```python
from build123d import *

# Parameters (mm, degrees)
F0_W      = 60
F0_H      = 60
F0_R      = 1.665
F1_DEPTH  = 5
F2_W      = 60
F2_H      = 20
F3_DEPTH  = 5
F5_DEPTH  = 5
F7_R      = 1.945
F8_DEPTH  = 5
F9_R      = 12.55
F10_DEPTH = 2


with BuildPart() as f1:
    # F0 (on Top) → F1 (new body)
    with BuildSketch(Plane.XY):
        Rectangle(F0_W, F0_H)
        with Locations((-15, -15)):
            Circle(F0_R, mode=Mode.SUBTRACT)
        with Locations((15, -15)):
            Circle(F0_R, mode=Mode.SUBTRACT)
        with Locations((-15, 15)):
            Circle(F0_R, mode=Mode.SUBTRACT)
        with Locations((15, 15)):
            Circle(F0_R, mode=Mode.SUBTRACT)
    extrude(amount=F1_DEPTH)

    # F2 (on face) → F3 (join)
    with BuildSketch(Plane.XZ.offset(30)):
        with Locations((0, -5)):
            Rectangle(F2_W, F2_H)
    extrude(amount=F3_DEPTH)

    # F4 (on face) → F5 (join)
    with BuildSketch(Plane.YZ.offset(30)):
        Polygon((-30, -15), (30, 0), (30, 5), (-35, 5), (-35, -15), align=None)
    extrude(amount=F5_DEPTH)

    # F6: F1 across plane


with BuildPart() as f1_1:
    add(f1.part)
    add(f1.part.mirror(Plane.YZ))

    # F7 (on face) → F8 (cut, through all)
    with BuildSketch(Plane.XZ.offset(35)):
        with Locations((-25, -5)):
            Circle(F7_R)
        with Locations((25, -5)):
            Circle(F7_R)
    extrude(amount=-F8_DEPTH, mode=Mode.SUBTRACT)

    # F9 (on face) → F10 (cut)
    with BuildSketch(Plane.XY.offset(5)):
        with Locations((0, 3.7)):
            Circle(F9_R)
    extrude(amount=-F10_DEPTH, mode=Mode.SUBTRACT)


solid = f1_1.part
```
Input: part model. Units: mm. Frame: model coordinates. A direction names the side the tool comes from. Round coordinates to 2 decimals unless told otherwise and drop trailing zeros. Write each loop counter-clockwise with the first axis right and the second up, starting at its lowest first coordinate (ties: lowest second). Pieces come first, ordered by that corner, then holes. Notation, with made-up numbers: (45, 18) - (89, 18) arc R18 cw to (89, 50) - close; hole circle Ø9 at (37, 27.5). An arc over 180 degrees is marked (long way). Write item = value, one per line.
(1) Section query C-C on z = -9.25. Output: boundary loops of the cut face in (x, y).
Geometry check:
outline = (-35, -35) - (35, -35) - (35, -7) - (30, -7) - (30, -30) - (-30, -30) - (-30, -7) - (-35, -7) - close
(2) Section query A-A on x = -25. Output: boundary loops of the cut face in (y, z) (3 decimals), then the cut area to 3 significant figures.
Geometry check:
outline = (-35, -15) - (-30, -15) - (-30, -6.945) - (-35, -6.945) - close; (-35, -3.055) - (-30, -3.055) - (-30, 0) - (30, 0) - (30, 5) - (-35, 5) - close
area = 381 mm^2
(3) Contact query for flat-ended pins moving along their axis: pin 1 Ø4 at (x, y) = (-15, -15) entering from -Z; pin 2 Ø4 at (x, y) = (-1, -6) entering from +Z; pin 3 Ø4.5 at (x, z) = (13.5, -9) entering from +Y. Output: stop coordinate, or through.
Geometry check:
pin_1 = 0
pin_2 = 3
pin_3 = -30
(4) Pull-direction query (X, two-part tool) for faces 1 (the flat face through (0, -33, -15)), 2 (the flat face through (35, -10, -3)), 3 (the cylindrical face through (16.538, -15.638, 2.465)); classes: +X half, -X half, draft (parallel to the pull), parting line (faces both ways), or undercut.
Geometry check:
face_1 = draft
face_2 = +X half
face_3 = undercut
(5) Section query B-B on x = 15. Output: boundary loops of the cut face in (y, z) (3 decimals).
Geometry check:
outline = (-35, -15) - (-30, -15) - (-30, 0) - (-16.665, 0) - (-16.665, 5) - (-35, 5) - close; (-13.335, 0) - (13.335, 0) - (13.335, 5) - (-13.335, 5) - close; (16.665, 0) - (30, 0) - (30, 5) - (16.665, 5) - close
(6) Material intervals for probe 1 along Y at (x, z) = (-15, 2.95) (3 decimals); probe 2 along X at (y, z) = (15, 2.75) (3 decimals); probe 3 along X at (y, z) = (6.5, -3.25), sorted ascending.
Geometry check:
probe_1 = -35 to -16.665, -13.335 to 13.335, 16.665 to 30
probe_2 = -35 to -16.665, -13.335 to 13.335, 16.665 to 35
probe_3 = -35 to -30, 30 to 35
(7) Section query D-D on y = -11. Output: boundary loops of the cut face in (x, z), then the cut area to 4 significant figures.
Geometry check:
outline = (-35, -10.25) - (-30, -10.25) - (-30, 0) - (30, 0) - (30, -10.25) - (35, -10.25) - (35, 5) - (-35, 5) - close
area = 452.5 mm^2
(8) Access query for faces 4 (the flat face through (0, 4, 3)), 5 (the cylindrical face through (16.538, 14.362, 2.465)), 6 (the flat face through (0, -30, -7)). Directions: +Z, -Z, +X, -X, +Y, -Y. A direction counts if a zero-diameter tool reaches every point of the face in a straight line with its end or side. Return the directions, or none.
Geometry check:
face_4 = +Z
face_5 = +Z, -Z
face_6 = -Z, +Y
